```python
from build123d import *

# Parameters (mm, degrees)
EXTRUDE_1_DEPTH     = 6.35
SKETCH_2_R          = 1.5
CUT_EXTRUDE_1_DEPTH = 7.35


with BuildPart() as part:
    # 草图1 → 凸台-拉伸1 (new body)
    with BuildSketch(Plane(origin=(0, 0, 0), x_dir=(1, 0, 0), z_dir=(0, 1, 0))):
        with BuildLine():
            Line((-64.584796248, 56.678842543), (-64.584796248, -223.321157457))
            ThreePointArc((-64.584796248, -223.321157457), (-61.65586406, -230.392225269), (-54.584796248, -233.321157457))
            Line((-54.584796248, -233.321157457), (155.415203752, -233.321157457))
            ThreePointArc((155.415203752, -233.321157457), (162.486271564, -230.392225269), (165.415203752, -223.321157457))
            Line((165.415203752, -223.321157457), (165.415203752, 56.678842543))
            ThreePointArc((165.415203752, 56.678842543), (162.486271564, 63.749910354), (155.415203752, 66.678842543))
            Line((155.415203752, 66.678842543), (-54.584796248, 66.678842543))
            ThreePointArc((-54.584796248, 66.678842543), (-61.65586406, 63.749910354), (-64.584796248, 56.678842543))
        make_face()
    extrude(amount=EXTRUDE_1_DEPTH)

    # 草图2 → 切除-拉伸1 (cut, through all)
    with BuildSketch(Plane(origin=(0, 6.35, 0), x_dir=(1, 0, 0), z_dir=(0, 1, 0))):
        with Locations((68.915203752, -64.821157457)):
            Circle(SKETCH_2_R)
        with Locations((68.915203752, -101.821157457)):
            Circle(SKETCH_2_R)
        with Locations((31.915203752, -101.821157457)):
            Circle(SKETCH_2_R)
        with Locations((31.915203752, -64.821157457)):
            Circle(SKETCH_2_R)
        with Locations((111.415203752, -48.821157457)):
            Circle(SKETCH_2_R)
        with Locations((154.415203752, -48.821157457)):
            Circle(SKETCH_2_R)
        with Locations((111.415203752, -117.821157457)):
            Circle(SKETCH_2_R)
        with Locations((154.415203752, -117.821157457)):
            Circle(SKETCH_2_R)
        with Locations((-53.584796248, -117.821157457)):
            Circle(SKETCH_2_R)
        with Locations((-10.584796248, -117.821157457)):
            Circle(SKETCH_2_R)
        with Locations((-53.584796248, -48.821157457)):
            Circle(SKETCH_2_R)
        with Locations((-10.584796248, -48.821157457)):
            Circle(SKETCH_2_R)
        with Locations((28.915203752, -222.821157457)):
            Circle(SKETCH_2_R)
        with Locations((28.915203752, -153.821157457)):
            Circle(SKETCH_2_R)
        with Locations((71.915203752, -222.821157457)):
            Circle(SKETCH_2_R)
        with Locations((71.915203752, -153.821157457)):
            Circle(SKETCH_2_R)
        with Locations((71.915203752, 56.178842543)):
            Circle(SKETCH_2_R)
        with Locations((28.915203752, 56.178842543)):
            Circle(SKETCH_2_R)
        with Locations((71.915203752, -12.821157457)):
            Circle(SKETCH_2_R)
        with Locations((28.915203752, -12.821157457)):
            Circle(SKETCH_2_R)
        with Locations((127.665203752, -146.791157457)):
            Circle(SKETCH_2_R)
        with Locations((158.945203752, -164.851157457)):
            Circle(SKETCH_2_R)
        with Locations((158.945203752, -1.791157457)):
            Circle(SKETCH_2_R)
        with Locations((127.665203752, -19.851157457)):
            Circle(SKETCH_2_R)
        with Locations((-58.114796248, -1.791157457)):
            Circle(SKETCH_2_R)
        with Locations((-26.834796248, -19.851157457)):
            Circle(SKETCH_2_R)
        with Locations((-58.114796248, -164.851157457)):
            Circle(SKETCH_2_R)
        with Locations((-26.834796248, -146.791157457)):
            Circle(SKETCH_2_R)
        with BuildLine():
            Line((30.415203752, -124.071157457), (70.415203752, -124.071157457))
            ThreePointArc((70.415203752, -124.071157457), (76.415203752, -118.071157457), (70.415203752, -112.071157457))
            Line((70.415203752, -112.071157457), (30.415203752, -112.071157457))
            ThreePointArc((30.415203752, -112.071157457), (24.415203752, -118.071157457), (30.415203752, -124.071157457))
        make_face()
        with BuildLine():
            Line((30.415203752, -42.571157457), (70.415203752, -42.571157457))
            ThreePointArc((70.415203752, -42.571157457), (76.415203752, -48.571157457), (70.415203752, -54.571157457))
            Line((70.415203752, -54.571157457), (30.415203752, -54.571157457))
            ThreePointArc((30.415203752, -54.571157457), (24.415203752, -48.571157457), (30.415203752, -42.571157457))
        make_face()
        with BuildLine():
            Line((12.915203752, -63.321157457), (12.915203752, -103.321157457))
            ThreePointArc((12.915203752, -103.321157457), (6.915203752, -109.321157457), (0.915203752, -103.321157457))
            Line((0.915203752, -103.321157457), (0.915203752, -63.321157457))
            ThreePointArc((0.915203752, -63.321157457), (6.915203752, -57.321157457), (12.915203752, -63.321157457))
        make_face()
        with BuildLine():
            Line((87.915203752, -63.321157457), (87.915203752, -103.321157457))
            ThreePointArc((87.915203752, -103.321157457), (93.915203752, -109.321157457), (99.915203752, -103.321157457))
            Line((99.915203752, -103.321157457), (99.915203752, -63.321157457))
            ThreePointArc((99.915203752, -63.321157457), (93.915203752, -57.321157457), (87.915203752, -63.321157457))
        make_face()
    extrude(amount=-CUT_EXTRUDE_1_DEPTH, mode=Mode.SUBTRACT)


solid = part.part
```
Check sheet for the modelled part. Datum: model origin and axes. Units: mm. A direction names the side the tool comes from. Give positions to 0.01 mm unless a question says otherwise; leave off trailing zeros. Write each loop counter-clockwise with the first axis right and the second up, starting at its lowest first coordinate (ties: lowest second). Pieces come first, ordered by that corner, then holes. Notation, with made-up numbers: (1, 4.25) - (28, 4.25) arc R36 ccw to (28, 41.25) - close; hole circle Ø1 at (26, 76.25). An arc over 180 degrees is marked (long way). Answer as a JSON object with one key per item and string values. Group by question number.
1) Sectioned sample at A-A (x = 63). Record the cut outline in (y, z).
2) Release check for a two-part mould opening along Z. For faces 1 (the face through (162.41, 3.13, 230.47)), 2 (the face through (24.417, 3.219, 48.703)), 3 (the face through (49, 0, 81)) record: pulls with the +Z half, pulls with the -Z half, needs draft (parallel to the pull), parting line crosses it, or undercut.
3) Thickness scan on probe 1 along Z at (x, y) = (127.5, 4.75); probe 2 along X at (y, z) = (4.5, 65); probe 3 along Z at (x, y) = (50, 3.25). Record the ranges inside material, lowest first. Write a range as from..to.
4) Access from +Z, -Z, +X, -X, +Y, -Y to the whole of each face (thin tool, end or side, straight path). Record for faces 4 (the face through (6.783, 3.219, 57.323)), 5 (the face through (49, 6.35, 81)).
5) Sectioned sample at B-B (y = 2). Give the number of separate pieces and of enclosed holes in the cut face, then the cut area to 3 significant figures.
Geometry results:
{
 "1": {"outline": "(0, -66.68) - (6.35, -66.68) - (6.35, 42.57) - (0, 42.57) - close; (0, 54.57) - (6.35, 54.57) - (6.35, 112.07) - (0, 112.07) - close; (0, 124.07) - (6.35, 124.07) - (6.35, 233.32) - (0, 233.32) - close"},
 "2": {"face 1": "pulls with the +Z half", "face 2": "undercut", "face 3": "needs draft"},
 "3": {"probe 1": "z = -66.68..18.36, 21.34..145.3, 148.28..233.32", "probe 2": "x = -64.58..0.92, 12.92..30.43, 33.4..67.43, 70.4..87.92, 99.92..165.42", "probe 3": "z = -66.68..42.57, 54.57..112.07, 124.07..233.32"},
 "4": {"face 4": "+Y, -Y", "face 5": "+Z, -Z, +X, -X, +Y"},
 "5": {"separate pieces": "1", "enclosed holes": "32", "area": "66,300 mm^2"}
}
